Could you check a few things on this model? Use its own coordinates, in mm. Face numbers are marked on the shaded views. A direction names the side the tool comes from. Round coordinates to 2 decimals unless told otherwise and drop trailing zeros. Loops run counter-clockwise (first coordinate to the right, second up) from the corner with the lowest first, then second, coordinate; pieces in that order, holes last. Notation, with made-up numbers: (9, 5) -> (32, 5) arc R23 ccw to (32, 29) -> close; hole circle Ø7 at (48.25, 67.25). An arc over 180 degrees is marked (long way). Write each question's results on one line, items separated by ' | '. Start each with the question number.
1) Imagine slicing it at C-C, the plane z = 0. List the corners of the cut face in (x, y) for me, plus the area to 3 significant figures.
2) Imagine slicing it at D-D, the plane x = 0. List the corners of the cut face in (y, z) for me.
3) Imagine slicing it at A-A, the plane y = 15. List the corners of the cut face in (x, z) for me, plus the area to 3 significant figures.
4) For P1, Ø3, axis at x = 3, z = 5, coming from the -Y side; P2, Ø5, axis at x = -1, z = 0, coming from the +Y side; P3, Ø3.5, axis at x = 0, z = 0, coming from the +Y side, each with a flat end and sliding along its axis, tell me the tip position at first contact or that it passes through.
5) If I drill on probe 1 along X at (y, z) = (15, -8.05); probe 2 along Y at (x, z) = (0, -7.35); probe 3 along X at (y, z) = (2.45, 0), over which ranges is the centre line in solid material (lowest first)?
6) Which directions (+Z, -Z, +X, -X, +Y, -Y) give clear straight access to the entire face, cutting with the end or side of a thin tool? Please do the marked faces 5 and 6.
7) Imagine slicing it at B-B, the plane y = 12.5. List the corners of the cut face in (x, z) for me, plus the area to 3 significant figures.
8) We'd pull the mould along X, two halves only. Please class the marked faces 1, 2, 3 and 4: pulls with the +X half, pulls with the -X half, needs draft (parallel to the pull), parting line crosses it, or undercut.
from build123d import *

# Parameters (mm, degrees)
SKETCH_1_W          = 10
SKETCH_1_H          = 18
SKETCH_1_R          = 3
EXTRUDE_2_DEPTH     = 4
SKETCH_3_W          = 10
SKETCH_3_H          = 3
EXTRUDE_3_DEPTH     = 16
SKETCH_4_R          = 2
CUT_EXTRUDE_1_DEPTH = 19
SKETCH_6_W          = 10
SKETCH_6_H          = 14.9
CUT_EXTRUDE_2_DEPTH = 1


with BuildPart() as part:
    # 草图1 → 凸台-拉伸2 (new body)
    with BuildSketch(Plane(origin=(0, 0, 0), x_dir=(1, 0, 0), z_dir=(0, 1, 0))):
        Rectangle(SKETCH_1_W, SKETCH_1_H)
        Circle(SKETCH_1_R, mode=Mode.SUBTRACT)
    extrude(amount=EXTRUDE_2_DEPTH)

    # 草图3 → 凸台-拉伸3 (add)
    with BuildSketch(Plane(origin=(0, 4, 0), x_dir=(1, 0, 0), z_dir=(0, 1, 0))):
        with Locations((0, -7.5)):
            Rectangle(SKETCH_3_W, SKETCH_3_H)
    extrude_3 = extrude(amount=EXTRUDE_3_DEPTH)

    # 草图4 → 切除-拉伸1 (cut, through all)
    with BuildSketch(Plane.XY.offset(9)):
        with Locations((0, 15)):
            Circle(SKETCH_4_R)
    cut_extrude_1 = extrude(amount=-CUT_EXTRUDE_1_DEPTH, mode=Mode.SUBTRACT)

    # 镜向1: 凸台-拉伸3, 切除-拉伸1 across plane
    add(extrude_3.mirror(Plane.XY))
    add(cut_extrude_1.mirror(Plane.XY), mode=Mode.SUBTRACT)

    # 草图6 → 切除-拉伸2 (cut)
    with BuildSketch(Plane.XZ):
        with Locations((0, 1.55)):
            Rectangle(SKETCH_6_W, SKETCH_6_H)
    extrude(amount=-CUT_EXTRUDE_2_DEPTH, mode=Mode.SUBTRACT)


solid = part.part
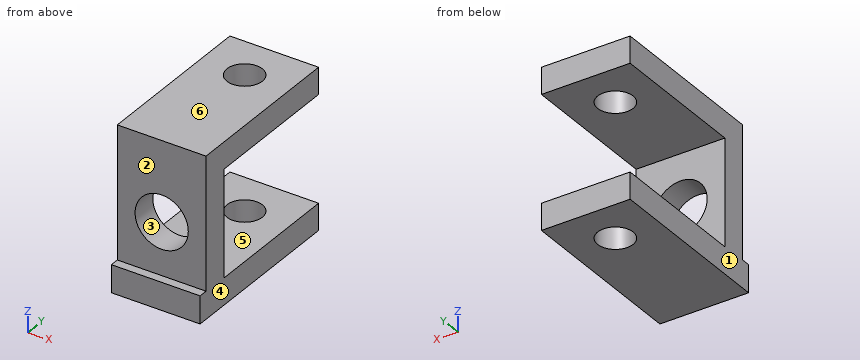
Checked values:
1) outline: (-5, 1) -> (-3, 1) -> (-3, 4) -> (-5, 4) -> close; (3, 1) -> (5, 1) -> (5, 4) -> (3, 4) -> close | area: 12.0 mm^2
2) outline: (0, -9) -> (13, -9) -> (13, -6) -> (4, -6) -> (4, -3) -> (1, -3) -> (1, -5.9) -> (0, -5.9) -> close; (1, 3) -> (4, 3) -> (4, 6) -> (13, 6) -> (13, 9) -> (1, 9) -> close; (17, -9) -> (20, -9) -> (20, -6) -> (17, -6) -> close; (17, 6) -> (20, 6) -> (20, 9) -> (17, 9) -> close
3) outline: (-5, -9) -> (-2, -9) -> (-2, -6) -> (-5, -6) -> close; (-5, 6) -> (-2, 6) -> (-2, 9) -> (-5, 9) -> close; (2, -9) -> (5, -9) -> (5, -6) -> (2, -6) -> close; (2, 6) -> (5, 6) -> (5, 9) -> (2, 9) -> close | area: 36.0 mm^2
4) P1: y = 1 | P2: y = 4 | P3: through
5) probe 1: -5 to -2, 2 to 5 | probe 2: 0 to 13, 17 to 20 | probe 3: -5 to -3, 3 to 5
6) face 5: +X, -X, +Y | face 6: +Z, +X, -X, +Y, -Y
7) outline: (-5, -9) -> (5, -9) -> (5, -6) -> (-5, -6) -> close; (-5, 6) -> (5, 6) -> (5, 9) -> (-5, 9) -> close | area: 60.0 mm^2
8) face 1: pulls with the -X half | face 2: needs draft | face 3: undercut | face 4: pulls with the +X half
